```python
from build123d import *

# Parameters (mm, degrees)
SKETCH1_R           = 2.1
BOSS_EXTRUDE1_DEPTH = 12
FILLET1_R           = 1
CUT_EXTRUDE1_DEPTH  = 12
FILLET3_R           = 0.25
FILLET4_R           = 3
BOSS_EXTRUDE2_DEPTH = 3
FILLET5_R           = 3
SKETCH7_R           = 3.5
CUT_EXTRUDE4_DEPTH  = 3


with BuildPart() as part:
    # Sketch1 → Boss-Extrude1 (new body)
    with BuildSketch(Plane.XY):
        with BuildLine():
            Line((12.5, 5.75), (12.5, -1.75))
            Line((12.5, -1.75), (3.707762128, -1.75))
            ThreePointArc((3.707762128, -1.75), (2.194880407, -3.463018914), (0, -4.1))
            Line((0, -4.1), (-20.5, -4.1))
            Line((-20.5, -4.1), (-20.5, -0.6))
            Line((-20.5, -0.6), (-4.055859958, -0.6))
            ThreePointArc((-4.055859958, -0.6), (-1.187820704, 3.924166405), (3.707762128, 1.75))
            Line((3.707762128, 1.75), (9, 1.75))
            Line((9, 1.75), (9, 5.75))
            Line((9, 5.75), (12.5, 5.75))
        make_face()
        Circle(SKETCH1_R, mode=Mode.SUBTRACT)
    extrude(amount=BOSS_EXTRUDE1_DEPTH)

    # Fillet1
    fillet1_edges = [part.edges().sort_by_distance(p)[0] for p in [
        (3.707762128, -1.75, 6),
        (12.5, -1.75, 6),
        (9, 1.75, 6),
        (3.707762128, 1.75, 6),
        (-4.055859958, -0.6, 6),
    ]]
    fillet(fillet1_edges, radius=FILLET1_R)

    # Sketch3 → Cut-Extrude1 (cut)
    with BuildSketch(Plane.XY.offset(12)):
        Polygon((9, 5.75), (12.5, 5.75), (12.5, 3.75), align=None)
    extrude(amount=-CUT_EXTRUDE1_DEPTH, mode=Mode.SUBTRACT)

    # Fillet3
    fillet3_edges = [part.edges().sort_by_distance(p)[0] for p in [
        (9, 5.75, 6),
    ]]
    fillet(fillet3_edges, radius=FILLET3_R)

    # Fillet4
    fillet4_edges = [part.edges().sort_by_distance(p)[0] for p in [
        (-20.5, -2.35, 0),
        (-20.5, -2.35, 12),
    ]]
    fillet(fillet4_edges, radius=FILLET4_R)

    # Sketch6 → Boss-Extrude2 (add)
    with BuildSketch(Plane.XZ.offset(4.1)):
        with BuildLine():
            Line((-8.5, 12), (-8.5, 0))
            Line((-8.5, 0), (-17.5, 0))
            ThreePointArc((-17.5, 0), (-19.621320344, 0.878679656), (-20.5, 3))
            Line((-20.5, 3), (-20.5, 9))
            ThreePointArc((-20.5, 9), (-19.621320344, 11.121320344), (-17.5, 12))
            Line((-17.5, 12), (-8.5, 12))
        make_face()
    extrude(amount=BOSS_EXTRUDE2_DEPTH)

    # Fillet5
    fillet5_edges = [part.edges().sort_by_distance(p)[0] for p in [
        (-8.5, -5.6, 0),
        (-8.5, -5.6, 12),
    ]]
    fillet(fillet5_edges, radius=FILLET5_R)

    # Sketch7 → Cut-Extrude4 (cut)
    with BuildSketch(Plane(origin=(0, -0.6, 0), x_dir=(1, 0, 0), z_dir=(0, 1, 0))):
        with Locations(Location((-14.5, -6, 0), (0, 0, 180))):
            Circle(SKETCH7_R)
    extrude(amount=-CUT_EXTRUDE4_DEPTH, mode=Mode.SUBTRACT)


solid = part.part
```
Check sheet for the modelled part. Datum: model origin and axes. Units: mm. A direction names the side the tool comes from. Give positions to 0.01 mm unless a question says otherwise; leave off trailing zeros. Write each loop counter-clockwise with the first axis right and the second up, starting at its lowest first coordinate (ties: lowest second). Pieces come first, ordered by that corner, then holes.
Item 1: Draft check along X on faces 1 (the face through (-19.6, -3.8, 0.86)), 2 (the face through (-1.066, 3.959, 5.916)), 3 (the face through (-9, -0.6, 6)), 4 (the face through (8.715, 2.051, 6.084)). Enter one of: released by +X, released by -X, zero draft, split by the parting line, or undercut.
Item 2: Cross-section at B-B (y = 0). Enter the section's corners in (x, z).
Item 3: Cross-section at D-D (z = 10.5). Enter the section's corners in (x, y).
Item 4: Cross-section at A-A (z = 6). Enter the section's corners in (x, y).
Item 5: Access from +Z, -Z, +X, -X, +Y, -Y to the whole of each face (thin tool, end or side, straight path). Record for faces 5 (the face through (-8.5, -6, 6)), 6 (the face through (9, 4, 6)), 7 (the face through (-9.36, -5.62, 11.1)).
Item 6: Scan lines: L1, parallel to Z at x = -14.5, y = -1.25; L2, parallel to X at y = -1, z = 3; L3, parallel to Y at x = 0, z = 9.25. Record each from-to range of solid material in increasing order.
Item 7: Gauge pin test, flat ends, axial feed: pin 1 (3.5 mm diameter, centred on x = -13, z = 5, fed in from +Y); pin 2 (3 mm diameter, centred on x = 6.5, z = 6.5, fed in from +Y); pin 3 (0.8 mm diameter, centred on y = 3.5, z = 8.5, fed in from -X); pin 4 (5 mm diameter, centred on x = 0, y = 0, fed in from +Z). Record the tip position at first contact, or that the pin passes through.
Item 8: Cross-section at C-C (x = -14.5). Enter the section's corners in (y, z).
Report:
1. face 1: released by -X
1. face 2: undercut
1. face 3: zero draft
1. face 4: undercut
2. outline: (-4.17, 0) - (-2.1, 0) - (-2.1, 12) - (-4.17, 12) - close; (2.1, 0) - (12.5, 0) - (12.5, 12) - (2.1, 12) - close
3. outline: (-20.1, -7.1) - (-8.9, -7.1) - (-8.9, -4.1) - (0, -4.1) arc R4.1 ccw to (3.45, -2.21) arc R1 cw to (4.3, -1.75) - (11.5, -1.75) arc R1 ccw to (12.5, -0.75) - (12.5, 3.75) - (9.37, 5.54) arc R0.25 ccw to (9, 5.32) - (9, 2.75) arc R1 cw to (8, 1.75) - (4.3, 1.75) arc R1 cw to (3.45, 2.21) arc R4.1 ccw to (-4.09, 0.32) arc R1 cw to (-5.08, -0.6) - (-20.1, -0.6) - close; hole circle Ø4.2 at (0, 0)
4. outline: (-20.5, -7.1) - (-8.5, -7.1) - (-8.5, -4.1) - (0, -4.1) arc R4.1 ccw to (3.45, -2.21) arc R1 cw to (4.3, -1.75) - (11.5, -1.75) arc R1 ccw to (12.5, -0.75) - (12.5, 3.75) - (9.37, 5.54) arc R0.25 ccw to (9, 5.32) - (9, 2.75) arc R1 cw to (8, 1.75) - (4.3, 1.75) arc R1 cw to (3.45, 2.21) arc R4.1 ccw to (-4.09, 0.32) arc R1 cw to (-5.08, -0.6) - (-11, -0.6) - (-11, -3.6) - (-18, -3.6) - (-18, -0.6) - (-20.5, -0.6) - close; hole circle Ø4.2 at (0, 0)
5. face 5: +Z, -Z, +X, -Y
5. face 6: +Z, -Z, +Y
5. face 7: +Z, +X, -Y
6. L1: z = 0 to 2.5, 9.5 to 12
6. L2: x = -20.5 to -16.3, -12.7 to -1.85, 1.85 to 12.47
6. L3: y = -4.1 to -2.1, 2.1 to 4.1
7. pin 1: stops at y = -0.6
7. pin 2: stops at y = 1.75
7. pin 3: stops at x = -2.68
7. pin 4: stops at z = 12
8. outline: (-7.1, 0) - (-0.6, 0) - (-0.6, 2.5) - (-3.6, 2.5) - (-3.6, 9.5) - (-0.6, 9.5) - (-0.6, 12) - (-7.1, 12) - close
